Solid Edge part; units mm, degrees
sketch "Sketch1" plane through (0, 0, 0) normal (0, -1, 0) x (1, 0, 0)
  line L0 (45.3, 43.3926) -> (45.3, 6.9074)
  line L1 (45.3, 6.9074) -> (39.3926, 1)
  line L2 (39.3926, 1) -> (19, 1)
  line L3 (19, 1) -> (15, -3)
  line L4 (15, -3) -> (0, -3)
  line L5 (0, 0) -> (0, -3)
  line L6 (13.7574, 0) -> (0, 0)
  line L7 (13.7574, 0) -> (17.7574, 4)
  line L8 (17.7574, 4) -> (38.15, 4)
  line L9 (42.3, 8.15) -> (38.15, 4)
  line L10 (42.3, 8.15) -> (42.3, 42.15)
  line L11 (42.3, 42.15) -> (38.15, 46.3)
  line L12 (17.7574, 46.3) -> (38.15, 46.3)
  line L13 (13.7574, 50.3) -> (17.7574, 46.3)
  line L14 (0, 50.3) -> (13.7574, 50.3)
  line L15 (0, 50.3) -> (0, 53.3)
  line L16 (0, 53.3) -> (15, 53.3)
  line L17 (15, 53.3) -> (19, 49.3)
  line L18 (19, 49.3) -> (39.3926, 49.3)
  line L19 (39.3926, 49.3) -> (45.3, 43.3926)
extrude "Protrusion1" add sketch "Sketch1" along normal blind 6
sketch "Sketch2" plane through (45.3, -3, 24.9165) normal (1, 0, 0) x (0, 0, -1)
  line L0 (-11.6335, 0.9) -> (11.1665, 0.9)
  line L1 (11.1665, 0.9) -> (11.1665, -0.9)
  line L2 (11.1665, -0.9) -> (-11.6335, -0.9)
  line L3 (-11.6335, -0.9) -> (-11.6335, 0.9)
extrude "VaciadoExtruido_1" cut sketch "Sketch2" against normal blind 3
sketch "Sketch3" plane through (45.3, -3, 24.9165) normal (1, 0, 0) x (0, 0, -1)
  line L0 (-13.7335, 3) -> (-13.7335, -3)
  line L1 (-13.7335, -3) -> (-10.0335, -3)
  line L2 (-10.0335, -3) -> (-10.0335, -0.9)
  line L3 (-10.0335, -0.9) -> (-11.6335, -0.9)
  line L4 (-11.6335, -0.9) -> (-11.6335, 0.9)
  line L5 (-11.6335, 0.9) -> (-10.0335, 0.9)
  line L6 (-10.0335, 0.9) -> (-10.0335, 3)
  line L7 (-10.0335, 3) -> (-13.7335, 3)
  line L8 (9.5665, -3) -> (9.5665, -0.9)
  line L9 (9.5665, -0.9) -> (11.1665, -0.9)
  line L10 (11.1665, -0.9) -> (11.1665, 0.9)
  line L11 (11.1665, 0.9) -> (9.5665, 0.9)
  line L12 (9.5665, 0.9) -> (9.5665, 3)
  line L13 (9.5665, 3) -> (13.2665, 3)
  line L14 (13.2665, 3) -> (13.2665, -3)
  line L15 (13.2665, -3) -> (9.5665, -3)
extrude "ProtrusiónExtruida_2" add sketch "Sketch3" along normal blind 19.8
sketch "Sketch4" plane through (0, -3, -1.5) normal (-1, 0, 0) x (0, 0, 1)
  line L0 (-7.6, 6) -> (-7.6, 0)
  line L1 (-4.4, 0) -> (-4.4, 6)
  arc A0 (-4.4, 0) -> (-7.6, 0) centre (-6, 0) cw
  arc A1 (-7.6, 6) -> (-4.4, 6) centre (-6, 6) cw
  line L2 (-1.5, -3) -> (-1.5, 9)
  line L3 (-1.5, 9) -> (-10.5, 9)
  line L4 (-10.5, 9) -> (-10.5, -3)
  line L5 (-10.5, -3) -> (-1.5, -3)
  line L6 (54.8, -3) -> (54.8, 9)
  line L7 (54.8, 9) -> (63.8, 9)
  line L8 (63.8, 9) -> (63.8, -3)
  line L9 (63.8, -3) -> (54.8, -3)
  arc A2 (60.9, 6) -> (57.7, 6) centre (59.3, 6) ccw
  line L10 (57.7, 0) -> (57.7, 6)
  arc A3 (57.7, 0) -> (60.9, 0) centre (59.3, 0) ccw
  line L11 (60.9, 6) -> (60.9, 0)
extrude "ProtrusiónExtruida_3" add sketch "Sketch4" against normal blind 3
fillet "Redondeo_1" radius 3 6 edges at (1.5, -6, 62.3) (1.5, 6, 62.3) (1.5, 6, 53.3) (1.5, 6, -12) (1.5, 6, -3) (1.5, -6, -12)
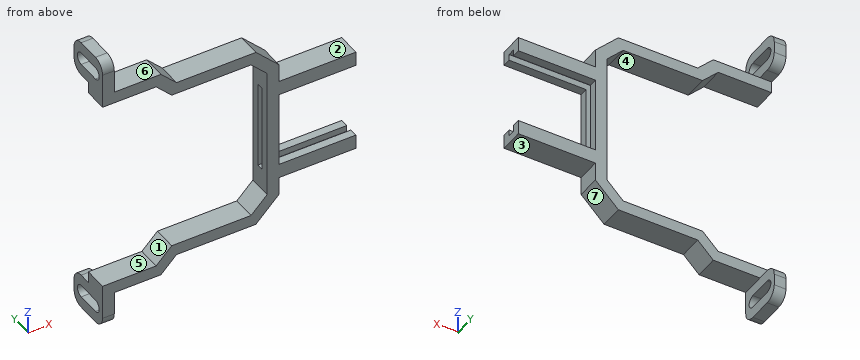
For this review, take the finished solid that the model builds, in its own axes (mm). Face numbers are marked on the shaded views. A direction names the side the tool comes from. Round coordinates to 2 decimals unless told otherwise and drop trailing zeros. Loops run counter-clockwise (first coordinate to the right, second up) from the corner with the lowest first, then second, coordinate; pieces in that order, holes last. Notation, with made-up numbers: (42.5, 24) - (77.5, 24) arc R18 cw to (77.5, 31) - close; hole circle Ø7 at (-5, 52.25). An arc over 180 degrees is marked (long way). Put each result on its own line as item: value. Start each with the question number.
1. Mouldability with a two-part tool opening along Z and no side actions: class the marked faces 4, 5, 6 and 7 as +Z half, -Z half, draft (parallel to the pull), parting line (faces both ways), or undercut.
2. For probe 1 along Z at (x, y) = (27, -1); probe 2 along Z at (x, y) = (5, -4); probe 3 along Y at (x, z) = (28, 47.5), list the stretches that pass through material, from the lowest coordinate up. Write a range as [from, to].
3. Insertion check: P1, Ø5, axis at x = 17, y = 1, coming from the -Z side; P2, Ø5, axis at y = -4, z = 23.5, coming from the -X side; P3, Ø5, axis at x = 27.5, y = -4.5, coming from the +Z side; P4, Ø4, axis at x = 20, z = -2.5, coming from the -Y side. Each pin has a flat end and moves straight along its axis. Give the tip position at first contact, or say it passes through.
4. Consider section D-D on x = 48. State the section outline as (y, z) points.
5. Consider section B-B on z = 57.8. State the section outline as (x, y) points.
6. Consider section A-A on y = 1. State the section outline as (x, z) points.
7. Consider section C-C on x = 9. State the section outline as (y, z) points.
8. For the marked faces 1, 2 and 3, list the 3-axis set-ups (+Z, -Z, +X, -X, +Y, -Y) from which the entire face can be reached by the end or side of a thin tool; tool diameter is ignored.
Result sheet:
1. face 4: undercut
1. face 5: undercut
1. face 6: +Z half
1. face 7: -Z half
2. probe 1: [1, 4], [46.3, 49.3]
2. probe 2: [-3, 0], [50.3, 53.3]
2. probe 3: [-6, 0]
3. P1: z = -3
3. P2: x = 42.3
3. P3: z = 49.3
3. P4: through
4. outline: (-6, 11.65) - (0, 11.65) - (0, 15.35) - (-2.1, 15.35) - (-2.1, 13.75) - (-3.9, 13.75) - (-3.9, 15.35) - (-6, 15.35) - close; (-6, 34.95) - (-3.9, 34.95) - (-3.9, 36.55) - (-2.1, 36.55) - (-2.1, 34.95) - (0, 34.95) - (0, 38.65) - (-6, 38.65) - close
5. outline: (0, -6) - (3, -6) - (3, -4.6) - (0, -4.6) - close; (0, 4.6) - (3, 4.6) - (3, 6) - (0, 6) - close
6. outline: (0, -12) - (3, -12) - (3, -9.1) - (0, -9.1) - close; (0, -5.9) - (3, -5.9) - (3, -3) - (0, -3) - close; (0, 53.3) - (3, 53.3) - (3, 56.2) - (0, 56.2) - close; (0, 59.4) - (3, 59.4) - (3, 62.3) - (0, 62.3) - close
7. outline: (-6, -3) - (0, -3) - (0, 0) - (-6, 0) - close; (-6, 50.3) - (0, 50.3) - (0, 53.3) - (-6, 53.3) - close
8. face 1: -X, +Y, -Y
8. face 2: +Z, +X, +Y, -Y
8. face 3: -Z, +X, +Y, -Y
